```python
from build123d import *

# Parameters (mm, degrees)
SKETCH4_R           = 25
BOSS_EXTRUDE2_DEPTH = 5
SKETCH5_R           = 10
CUT_EXTRUDE1_DEPTH  = 36.707142143
BOSS_EXTRUDE3_DEPTH = 3.75
SKETCH1_R           = 25
SKETCH1_R_2         = 15.5
CUT_EXTRUDE2_DEPTH  = 38.584072424


with BuildPart() as part:
    # Sketch4 → Boss-Extrude2 (new body)
    with BuildSketch(Plane.XY):
        Circle(SKETCH4_R)
    extrude(amount=BOSS_EXTRUDE2_DEPTH)

    # Sketch5 → Cut-Extrude1 (cut, through all)
    with BuildSketch(Plane.XY.offset(5)):
        Circle(SKETCH5_R)
    extrude(amount=-CUT_EXTRUDE1_DEPTH, mode=Mode.SUBTRACT)

    # Sketch6 → Boss-Extrude3 (add, symmetric)
    with BuildSketch(Plane(origin=(0, 0, 0), x_dir=(1, 0, 0), z_dir=(0, 1, 0))):
        Polygon((15.5, 12.75), (12.603553391, 12.75), (12, 12.146446609), (12, 10.207106781), (12.75, 9.457106781), (12.75, 2.396446609), (10.353553391, 0), (15.5, 0), align=None)
    boss_extrude3 = extrude(amount=BOSS_EXTRUDE3_DEPTH, both=True)

    # Sketch1 → Cut-Extrude2 (cut, through all)
    with BuildSketch(Plane.XY):
        Circle(SKETCH1_R)
        Circle(SKETCH1_R_2, mode=Mode.SUBTRACT)
    cut_extrude2 = extrude(amount=-CUT_EXTRUDE2_DEPTH, mode=Mode.SUBTRACT)

    # Sketch6_4 → Cut-Revolve1 (revolve, cut)
    with BuildSketch(Plane(origin=(0, 0, 0), x_dir=(1, 0, 0), z_dir=(0, 1, 0))):
        with BuildLine():
            add(Edge.make_bspline(
                [(14.75, 12.75), (14.75, 3.446446626), (15.5, 0)],
                knots=[0, 0, 0, 1, 1, 1], degree=2))
            Line((15.5, 0), (15.5, 12.75))
            Line((15.5, 12.75), (14.75, 12.75))
        make_face()
    cut_revolve1 = revolve(axis=Axis((0, 0, 0), (0, 0, -1)), mode=Mode.SUBTRACT)

    # Mirror1: Boss-Extrude3, Cut-Extrude2, Cut-Revolve1 across plane
    add(boss_extrude3.mirror(Plane(origin=(0, 0, 0), x_dir=(0, 0, 1), z_dir=(1, 0, 0))))
    add(cut_extrude2.mirror(Plane(origin=(0, 0, 0), x_dir=(0, 0, 1), z_dir=(1, 0, 0))), mode=Mode.SUBTRACT)
    add(cut_revolve1.mirror(Plane(origin=(0, 0, 0), x_dir=(0, 0, 1), z_dir=(1, 0, 0))), mode=Mode.SUBTRACT)


solid = part.part
```
Here's how the part is built. I have some questions about the finished solid (model axes, mm). A direction names the side the tool comes from. Give positions to 0.01 mm unless a question says otherwise; leave off trailing zeros. Order: outer loops, then holes, each group sorted by start corner. A loop starts at its lowest first (then second) coordinate and runs counter-clockwise, first axis right, second up. Notation, with made-up numbers: (-22, 64.25) - (-3, 64.25) arc R18 ccw to (-3, 93.25) - close; hole circle Ø9 at (24.5, 17). An arc over 180 degrees is marked (long way). Answer as a JSON object with one key per item and string values. Group by question number.
Item 1: If we section it at C-C on x = 8: Please give me the cut outline in (y, z), and give its area (3 significant figures).
Item 2: If we section it at B-B on y = 20: Please give me the cut outline in (x, z), and give its area (3 significant figures).
Item 3: If we mould it in two halves opening along Z, with no side actions, what happens to faces 1 (the cylindrical face through (-2.17, -9.76, 2.54)), 2 (the flat face through (11.569, 0.053, -1.215)), 3 (the flat face through (-14, 0, -12.75))? For each: pulls with the +Z half, pulls with the -Z half, needs draft (parallel to the pull), parting line crosses it, or undercut.
Item 4: Please list where these lines run through material, in increasing order: probe 1 along Y at (x, z) = (0, 2.6); probe 2 along Z at (x, y) = (14.5, 15); probe 3 along X at (y, z) = (2.5, -3.75).
Item 5: If we section it at D-D on x = 20.5: Please give me the cut outline in (y, z).
Item 6: For P1, Ø4, axis at y = 10.5, z = -2.5, coming from the +X side; P2, Ø6, axis at y = 3.5, z = -7, coming from the -X side; P3, Ø2, axis at y = 0, z = -5, coming from the -X side; P4, Ø0.6, axis at y = -1, z = -11.5, coming from the -X side, each with a flat end and sliding along its axis, tell me the tip position at first contact or that it passes through.
Item 7: Which directions (+Z, -Z, +X, -X, +Y, -Y) give clear straight access to the entire face, cutting with the end or side of a thin tool? Please do faces 4 (the flat face through (13, -3.75, -6)), 5 (the flat face through (-13, 3.75, -6)), 6 (the flat face through (12.75, 0, -6)).
Item 8: If we section it at A-A on x = 0: Please give me the cut outline in (y, z), and give its area (3 significant figures).
Result set:
{
 "1": {"outline": "(-23.69, 0) - (-6, 0) - (-6, 5) - (-23.69, 5) - close; (6, 0) - (23.69, 0) - (23.69, 5) - (6, 5) - close", "area": "177 mm²"},
 "2": {"outline": "(-15, 0) - (15, 0) - (15, 5) - (-15, 5) - close", "area": "150 mm²"},
 "3": {"face 1": "needs draft", "face 2": "undercut", "face 3": "pulls with the -Z half"},
 "4": {"probe 1": "-25 to -10, 10 to 25", "probe 2": "0 to 5", "probe 3": "-14.81 to -12.75, 12.75 to 14.81"},
 "5": {"outline": "(-14.31, 0) - (14.31, 0) - (14.31, 5) - (-14.31, 5) - close"},
 "6": {"P1": "through", "P2": "x = -14.88", "P3": "x = -15", "P4": "x = -14.74"},
 "7": {"face 4": "-Z, +X, -X, -Y", "face 5": "-Z, +X, -X, +Y", "face 6": "+Y, -Y"},
 "8": {"outline": "(-25, 0) - (-10, 0) - (-10, 5) - (-25, 5) - close; (10, 0) - (25, 0) - (25, 5) - (10, 5) - close", "area": "150 mm²"}
}
